Check sheet for the modelled part. Datum: model origin and axes. Units: mm. Give positions to 0.01 mm unless a question says otherwise; leave off trailing zeros. Answer in a Markdown table with one row per item. Add a question column.
(1) Draft check along Y on faces 1 (the face through (37.15, 0.01, 2.45)), 2 (the face through (38, 49, 6.35)), 3 (the face through (-3.63, -3.49, 3.13)), 4 (the face through (-3.49, 99.98, 3.13)). Enter one of: released by +Y, released by -Y, zero draft, split by the parting line, or undercut.
(2) Go/stop test with flat-tipped pins: P1, Ø3.5, axis at x = 38.17, y = 97.9, coming from the -Z side; P2, Ø5, axis at x = 38.17, y = -1.59, coming from the -Z side. Record where each tip stops, or that it passes through.
(3) Thickness scan on L1, parallel to X at y = 48, z = 5.25; L2, parallel to X at y = 49, z = 5; L3, parallel to Y at x = 78.5, z = 1.75. Record the ranges inside material, lowest first.
from build123d import *

# Parameters (mm, degrees)
SKETCH1_R                                         = 1.5875
BOSS_EXTRUDE1_DEPTH                               = 6.35
CSK_FOR_6_FLAT_HEAD_MACHINE_SCREW_100_D           = 3.7973
CSK_FOR_6_FLAT_HEAD_MACHINE_SCREW_100_CSINK_D     = 7.0866
CSK_FOR_6_FLAT_HEAD_MACHINE_SCREW_100_CSINK_ANGLE = 100


with BuildPart() as part:
    # Sketch1 → Boss-Extrude1 (new body)
    with BuildSketch(Plane.XY):
        with BuildLine():
            Line((3.175, -6.35), (73.174999954, -6.35))
            ThreePointArc((73.174999954, -6.35), (79.910192045, -3.560192091), (82.699999954, 3.175))
            Line((82.699999954, 3.175), (82.699999954, 93.175000086))
            ThreePointArc((82.699999954, 93.175000086), (79.910192045, 99.910192177), (73.174999954, 102.700000086))
            Line((73.174999954, 102.700000086), (3.175, 102.700000086))
            ThreePointArc((3.175, 102.700000086), (-3.560192091, 99.910192177), (-6.35, 93.175000086))
            Line((-6.35, 93.175000086), (-6.35, 3.175))
            ThreePointArc((-6.35, 3.175), (-3.560192091, -3.560192091), (3.175, -6.35))
        make_face()
        with Locations((38.174999977, -1.5875)):
            Circle(SKETCH1_R, mode=Mode.SUBTRACT)
        with Locations((77.937499954, 48.175000043)):
            Circle(SKETCH1_R, mode=Mode.SUBTRACT)
        with Locations((38.174999977, 97.937500086)):
            Circle(SKETCH1_R, mode=Mode.SUBTRACT)
        with Locations((-1.5875, 48.175000043)):
            Circle(SKETCH1_R, mode=Mode.SUBTRACT)
    extrude(amount=BOSS_EXTRUDE1_DEPTH)

    # CSK for #6 Flat Head Machine Screw (100)1 (through all)
    with Locations(Plane.XY.offset(6.35)):
        with Locations((-1.5875, 48.175000043), (77.937499954, 48.175000043), (38.174999977, -1.5875), (38.174999977, 97.900367712)):
            CounterSinkHole(CSK_FOR_6_FLAT_HEAD_MACHINE_SCREW_100_D / 2, CSK_FOR_6_FLAT_HEAD_MACHINE_SCREW_100_CSINK_D / 2, counter_sink_angle=CSK_FOR_6_FLAT_HEAD_MACHINE_SCREW_100_CSINK_ANGLE)


solid = part.part
Reply:
| question | item | result |
|---|---|---|
| 1 | face 1 | undercut |
| 1 | face 2 | zero draft |
| 1 | face 3 | released by -Y |
| 1 | face 4 | released by +Y |
| 2 | P1 | through |
| 2 | P2 | z = 0 |
| 3 | L1 | -6.35 to -3.81, 0.64 to 75.71, 80.16 to 82.7 |
| 3 | L2 | -6.35 to -3.34, 0.16 to 76.19, 79.69 to 82.7 |
| 3 | L3 | -4.72 to 46.36, 49.99 to 101.07 |
